Verification items for the finished model (mm, model axes). Face numbers are marked on the shaded views. A direction names the side the tool comes from. Give positions to 0.01 mm unless a question says otherwise; leave off trailing zeros. Loops run counter-clockwise (first coordinate to the right, second up) from the corner with the lowest first, then second, coordinate; pieces in that order, holes last. Notation, with made-up numbers: M 55,-14.75 L 82,-14.75 A15 cw 82,0.25 Z; hole C 83.5,-36 d3. An arc over 180 degrees is marked long. Use a Markdown table: item, result.
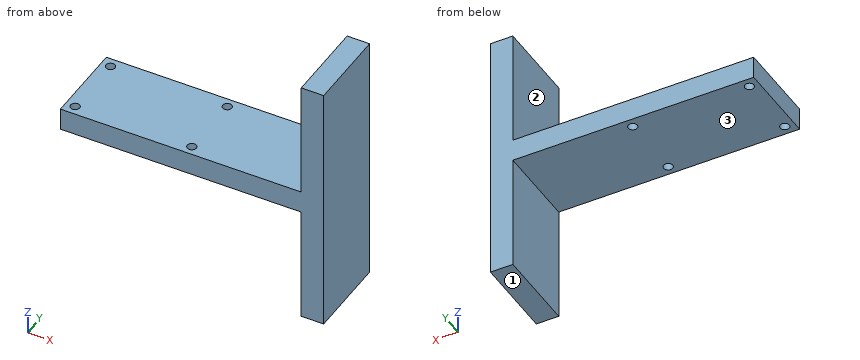
Solid Edge part; units mm, degrees
sketch "Sketch1" plane through (0, 0, 0) normal (0, 0, 1) x (1, 0, 0)
  line L0 (0, 0) -> (46.5, 0)
  line L1 (46.5, 0) -> (46.5, 28.5)
  line L2 (46.5, 28.5) -> (0, 28.5)
  line L3 (0, 28.5) -> (0, 0)
extrude "Protrusion1" add sketch "Sketch1" along normal blind 7.7
hole "Bohrung_1" at (3.25, 25.25, 7.7) direction (0, 0, -1) diameter 3.1 end up to next
hole "Hole1" at (43.25, 25.25, 7.7) direction (0, 0, -1) diameter 3.1 end up to next
hole "Hole2" at (43.25, 3.25, 7.7) direction (0, 0, -1) diameter 3.1 end up to next
hole "Hole3" at (3.25, 3.25, 7.7) direction (0, 0, -1) diameter 3.1 end up to next
sketch "Sketch2" plane through (46.5, 14.25, 3.85) normal (1, 0, 0) x (0, 1, 0)
  line L0 (-14.25, 3.85) -> (14.25, 3.85)
  line L1 (14.25, 3.85) -> (14.25, -3.85)
  line L2 (14.25, -3.85) -> (-14.25, -3.85)
  line L3 (-14.25, -3.85) -> (-14.25, 3.85)
extrude "Extrusionsausprägung_2" add sketch "Sketch2" along normal blind 36.05
sketch "Sketch3" plane through (82.55, 14.25, 3.85) normal (1, 0, 0) x (0, 1, 0)
  line L0 (14.25, 3.85) -> (14.25, 43.85)
  line L1 (14.25, 43.85) -> (-14.25, 43.85)
  line L2 (-14.25, 3.85) -> (-14.25, 43.85)
  line L3 (-14.25, 3.85) -> (-14.25, -3.85)
  line L4 (-14.25, -3.85) -> (-14.25, -43.85)
  line L5 (-14.25, -43.85) -> (14.25, -43.85)
  line L6 (14.25, -43.85) -> (14.25, 3.85)
  dimension "D1" = 14.25
extrude "Extrusionsausprägung_3" add sketch "Sketch3" along normal blind 7.7
(1) Cross-section at C-C on y = 15.75. Record the cut outline in (x, z).
Results below:
| item | result |
|---|---|
| outline | M 0,0 L 82.55,0 L 82.55,-40 L 90.25,-40 L 90.25,47.7 L 82.55,47.7 L 82.55,7.7 L 0,7.7 Z |
(2) Cross-section at B-B on y = 25.25. Record the cut outline in (x, z).
Results below:
| item | result |
|---|---|
| outline | M 0,0 L 1.7,0 L 1.7,7.7 L 0,7.7 Z; M 4.8,0 L 41.7,0 L 41.7,7.7 L 4.8,7.7 Z; M 44.8,0 L 82.55,0 L 82.55,-40 L 90.25,-40 L 90.25,47.7 L 82.55,47.7 L 82.55,7.7 L 44.8,7.7 Z |
(3) Cross-section at A-A on x = 43.25. Record the cut outline in (y, z).
Results below:
| item | result |
|---|---|
| outline | M 0,0 L 1.7,0 L 1.7,7.7 L 0,7.7 Z; M 4.8,0 L 23.7,0 L 23.7,7.7 L 4.8,7.7 Z; M 26.8,0 L 28.5,0 L 28.5,7.7 L 26.8,7.7 Z |
(4) Set-up check for the marked faces 1, 2 and 3: record each of +Z, -Z, +X, -X, +Y, -Y from which the full face is reachable in a straight line by a thin tool's end or side.
Results below:
| item | result |
|---|---|
| face 1 | -Z, +X, -X, +Y, -Y |
| face 2 | +Z, -X, +Y, -Y |
| face 3 | -Z, -X, +Y, -Y |
(5) Material ranges on line 1 (Y direction, x = 43.25, z = 5.25); line 2 (X direction, y = 25.25, z = 5); line 3 (X direction, y = 8.5, z = 38.5), recorded low to high.
Results below:
| item | result |
|---|---|
| line 1 | 0 to 1.7, 4.8 to 23.7, 26.8 to 28.5 |
| line 2 | 0 to 1.7, 4.8 to 41.7, 44.8 to 90.25 |
| line 3 | 82.55 to 90.25 |
(6) Gauge pin test, flat ends, axial feed: P1, Ø5, axis at x = 43.25, y = 3.25, coming from the -Z side; P2, Ø3, axis at x = 78.5, y = 21.5, coming from the +Z side; P3, Ø14, axis at y = 9.5, z = -25.5, coming from the -X side. Record the tip position at first contact, or that the pin passes through.
Results below:
| item | result |
|---|---|
| P1 | z = 0 |
| P2 | z = 7.7 |
| P3 | x = 82.55 |
(7) Cross-section at D-D on z = 13. Record the cut outline in (x, y).
Results below:
| item | result |
|---|---|
| outline | M 82.55,0 L 90.25,0 L 90.25,28.5 L 82.55,28.5 Z |
